Source: CAD feature listing. Evaluate the final solid. Frame: model axes, mm. Round coordinates to 2 decimals unless told otherwise and drop trailing zeros. Order: outer loops, then holes, each group sorted by start corner. A loop starts at its lowest first (then second) coordinate and runs counter-clockwise, first axis right, second up. Notation, with made-up numbers: (89.25, -32) -> (144.25, -32) arc R19 cw to (144.25, -22) -> close; hole circle Ø4 at (82, 22.5). An arc over 180 degrees is marked (long way). Answer as CSV lines item,"result". Start each with the question number.
(1) Contact query for a flat-ended pin moving along its axis: P1, Ø3, axis at x = -32.5, y = -23.25, coming from the +Z side. Output: stop coordinate, or through.
(2) Line query: line 1 along X through (y, z) = (-24.5, 0.85); line 2 along Y through (x, z) = (-11.5, 0.3); line 3 along Y through (x, z) = (32.5, 0.6). Output: solid intervals per line, ascending. Write a range as from..to.
(3) Section query A-A (z = 0.3). Output: boundary loops of the cut face in (x, y), plus the area to 3 significant figures.
(4) Section query C-C (y = 23.25). Output: boundary loops of the cut face in (x, z), plus the area to 3 significant figures.
(5) Section query B-B (x = 0). Output: boundary loops of the cut face in (y, z).
(6) Section query D-D (x = -32.5). Output: boundary loops of the cut face in (y, z).
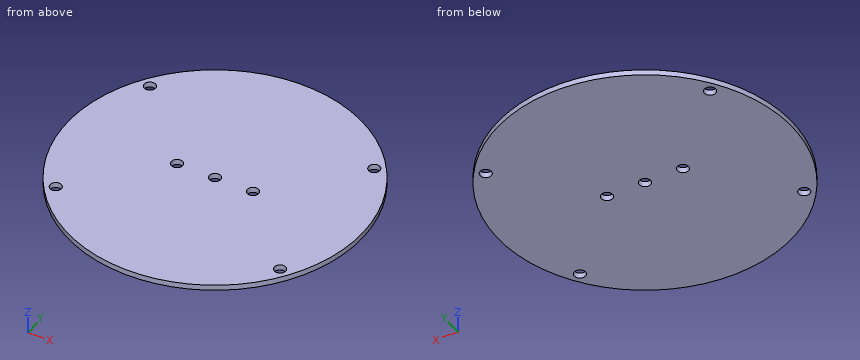
```python
from build123d import *

# Parameters (mm, degrees)
F0_R     = 43
F0_R_2   = 1.65
F0_R_3   = 25
F1_DEPTH = 1.6


with BuildPart() as f1:
    # F0 (on Top) → F1 (new body)
    with BuildSketch(Plane.XY):
        Circle(F0_R)
        with Locations((-32.5, -23.25)):
            Circle(F0_R_2, mode=Mode.SUBTRACT)
        with Locations((32.5, -23.25)):
            Circle(F0_R_2, mode=Mode.SUBTRACT)
        with Locations((-32.5, 23.25)):
            Circle(F0_R_2, mode=Mode.SUBTRACT)
        Circle(F0_R_3, mode=Mode.SUBTRACT)
        with Locations((32.5, 23.25)):
            Circle(F0_R_2, mode=Mode.SUBTRACT)
        Circle(F0_R_3)
        with Locations((-11, 0)):
            Circle(F0_R_2, mode=Mode.SUBTRACT)
        Circle(F0_R_2, mode=Mode.SUBTRACT)
        with Locations((11, 0)):
            Circle(F0_R_2, mode=Mode.SUBTRACT)
    extrude(amount=F1_DEPTH)


solid = f1.part
```
Answer block:
1,P1,"through"
2,line 1,"-35.34..-33.58, -31.42..31.42, 33.58..35.34"
2,line 2,"-41.43..-1.57, 1.57..41.43"
2,line 3,"-28.16..-24.9, -21.6..21.6, 24.9..28.16"
3,outline,"circle Ø86 at (0, 0); hole circle Ø3.3 at (-32.5, -23.25); hole circle Ø3.3 at (-32.5, 23.25); hole circle Ø3.3 at (-11, 0); hole circle Ø3.3 at (0, 0); hole circle Ø3.3 at (11, 0); hole circle Ø3.3 at (32.5, -23.25); hole circle Ø3.3 at (32.5, 23.25)"
3,area,"5,750 mm2"
4,outline,"(-36.17, 0) -> (-34.15, 0) -> (-34.15, 1.6) -> (-36.17, 1.6) -> close; (-30.85, 0) -> (30.85, 0) -> (30.85, 1.6) -> (-30.85, 1.6) -> close; (34.15, 0) -> (36.17, 0) -> (36.17, 1.6) -> (34.15, 1.6) -> close"
4,area,"105 mm2"
5,outline,"(-43, 0) -> (-1.65, 0) -> (-1.65, 1.6) -> (-43, 1.6) -> close; (1.65, 0) -> (43, 0) -> (43, 1.6) -> (1.65, 1.6) -> close"
6,outline,"(-28.16, 0) -> (-24.9, 0) -> (-24.9, 1.6) -> (-28.16, 1.6) -> close; (-21.6, 0) -> (21.6, 0) -> (21.6, 1.6) -> (-21.6, 1.6) -> close; (24.9, 0) -> (28.16, 0) -> (28.16, 1.6) -> (24.9, 1.6) -> close"
